Geometry: final body of the model. Coordinates: model frame, mm. Give positions to 0.01 mm unless a question says otherwise; leave off trailing zeros. Write each loop counter-clockwise with the first axis right and the second up, starting at its lowest first coordinate (ties: lowest second). Pieces come first, ordered by that corner, then holes. Notation, with made-up numbers: M 66,78.5 L 121,78.5 A6 cw 121,83.5 Z; hole C 54.5,44 d11. An arc over 180 degrees is marked long. Use a Markdown table: item, result. Add a question column.
1) Section A-A on z = -47.5. Return the cut outline in (x, y) (3 decimals), then the cut area to 3 significant figures.
2) Section C-C on y = -1.75. Return the cut outline in (x, z).
3) Line query: line 1 (X direction, y = -1.4, z = -72); line 2 (Z direction, x = -110.5, y = -2.3). Output: solid intervals per line, ascending.
4) Section B-B on x = 103. Return the cut outline in (y, z) (3 decimals).
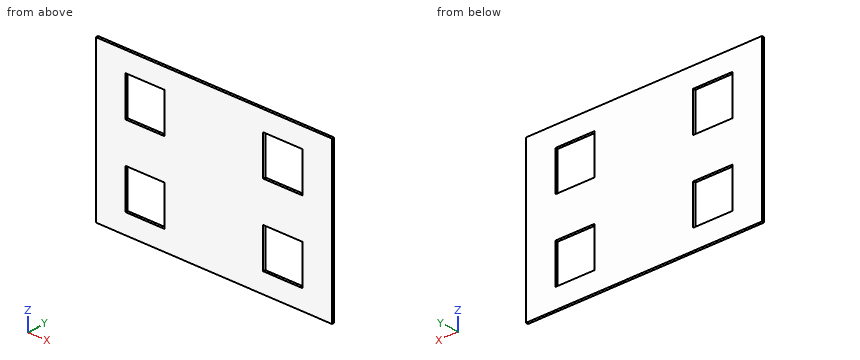
```python
from build123d import *

# Parameters (mm, degrees)
F0_W     = 50.8
F0_H     = 50.8
F1_DEPTH = 3.175


with BuildPart() as f1:
    # F0 (on Front) → F1 (new body)
    with BuildSketch(Plane.XZ):
        Polygon((152.4, 0), (152.4, 101.6), (0, 101.6), (-152.4, 101.6), (-152.4, 0), (-152.4, -101.6), (0, -101.6), (152.4, -101.6), align=None)
        with Locations((-88.9, -50.8)):
            Rectangle(F0_W, F0_H, mode=Mode.SUBTRACT)
        with Locations((88.9, -50.8)):
            Rectangle(F0_W, F0_H, mode=Mode.SUBTRACT)
        with Locations((-88.9, 50.8)):
            Rectangle(F0_W, F0_H, mode=Mode.SUBTRACT)
        with Locations((88.9, 50.8)):
            Rectangle(F0_W, F0_H, mode=Mode.SUBTRACT)
    extrude(amount=F1_DEPTH)


solid = f1.part
```
Found:
| question | item | result |
|---|---|---|
| 1 | outline | M -152.4,-3.175 L -114.3,-3.175 L -114.3,0 L -152.4,0 Z; M -63.5,-3.175 L 63.5,-3.175 L 63.5,0 L -63.5,0 Z; M 114.3,-3.175 L 152.4,-3.175 L 152.4,0 L 114.3,0 Z |
| 1 | area | 645 mm² |
| 2 | outline | M -152.4,-101.6 L 152.4,-101.6 L 152.4,101.6 L -152.4,101.6 Z; hole M -114.3,-76.2 L -63.5,-76.2 L -63.5,-25.4 L -114.3,-25.4 Z; hole M -114.3,25.4 L -63.5,25.4 L -63.5,76.2 L -114.3,76.2 Z; hole M 63.5,-76.2 L 114.3,-76.2 L 114.3,-25.4 L 63.5,-25.4 Z; hole M 63.5,25.4 L 114.3,25.4 L 114.3,76.2 L 63.5,76.2 Z |
| 3 | line 1 | -152.4 to -114.3, -63.5 to 63.5, 114.3 to 152.4 |
| 3 | line 2 | -101.6 to -76.2, -25.4 to 25.4, 76.2 to 101.6 |
| 4 | outline | M -3.175,-101.6 L 0,-101.6 L 0,-76.2 L -3.175,-76.2 Z; M -3.175,-25.4 L 0,-25.4 L 0,25.4 L -3.175,25.4 Z; M -3.175,76.2 L 0,76.2 L 0,101.6 L -3.175,101.6 Z |
